Could you check a few things on this model? Use its own coordinates, in mm. A direction names the side the tool comes from. Give positions to 0.01 mm unless a question says otherwise; leave off trailing zeros. Loops run counter-clockwise (first coordinate to the right, second up) from the corner with the lowest first, then second, coordinate; pieces in that order, holes last.
1. For faces 1 (the flat face through (0, 5, 0)), 2 (the flat face through (-9, 0, 91)), 3 (the flat face through (5.617, 5.423, 88.74)), which set-ups out of +Z, -Z, +X, -X, +Y, -Y let a thin tool reach every point of the face, with its end or its side?
2. Imagine slicing it at C-C (y = 3). List the corners of the cut face in (x, z) for me.
3. I need wall thicknesses on line 1 along Y through (x, z) = (-10, 23); line 2 along X through (y, z) = (9, 13.5); line 3 along X through (y, z) = (3.75, 53.5). Which ranges of each line are inside material? Lowest first, please.
4. Thinking about a two-plate mould opening in Y: for faces 4 (the flat face through (0, 5, 180)), 5 (the flat face through (9, 0, 91)), 6 (the flat face through (0, -2, 91)), 7 (the flat face through (-5.644, 5.577, 88.74)), which applies, +Y half, -Y half, draft (parallel to the pull), parting line (faces both ways), or undercut?
5. Imagine slicing it at B-B (x = -9). List the corners of the cut face in (y, z) for me.
6. Imagine slicing it at A-A (z = 83). List the corners of the cut face in (x, y) for me.
7. For P1, Ø12, axis at x = 8, z = 118, coming from the +Y side; P2, Ø3, axis at y = 6, z = 145, coming from the -X side; P3, Ø2, axis at y = 9, z = 137.5, coming from the +X side; P4, Ø1.5, axis at y = 7.5, z = 148.5, coming from the +X side, each with a flat end and sliding along its axis, tell me the tip position at first contact or that it passes through.
```python
from build123d import *

# Parameters (mm, degrees)
BOSS_EXTRUDE1_DEPTH = 180
SKETCH2_W           = 26
SKETCH2_H           = 180
BOSS_EXTRUDE2_DEPTH = 2


with BuildPart() as part:
    # Sketch1 → Boss-Extrude1 (new body)
    with BuildSketch(Plane.XY):
        Polygon((-6.6, 11), (-4.660403212, 0), (0, 0), (0, 11), align=None)
        Polygon((0, 11), (0, 0), (4.660403212, 0), (6.6, 11), align=None)
    extrude(amount=BOSS_EXTRUDE1_DEPTH)

    # Sketch2 → Boss-Extrude2 (add)
    with BuildSketch(Plane.XZ):
        with Locations((0, 90)):
            Rectangle(SKETCH2_W, SKETCH2_H)
    extrude(amount=BOSS_EXTRUDE2_DEPTH)


solid = part.part
```
Derived:
1. face 1: -Z, +X, -X, +Y, -Y
1. face 2: +Z, -Z, -X
1. face 3: +Z, -Z, +X
2. outline: (-5.19, 0) - (5.19, 0) - (5.19, 180) - (-5.19, 180) - close
3. line 1: y = -2 to 0
3. line 2: x = -6.25 to 6.25
3. line 3: x = -5.32 to 5.32
4. face 4: draft
4. face 5: undercut
4. face 6: -Y half
4. face 7: undercut
5. outline: (-2, 0) - (0, 0) - (0, 180) - (-2, 180) - close
6. outline: (-13, -2) - (13, -2) - (13, 0) - (4.66, 0) - (6.6, 11) - (-6.6, 11) - (-4.66, 0) - (-13, 0) - close
7. P1: stops at y = 11
7. P2: stops at x = -5.98
7. P3: stops at x = 6.42
7. P4: stops at x = 6.12
